```python
from build123d import *

# Parameters (mm, degrees)
SKETCH1_R           = 33.5
SKETCH1_R_2         = 4
BOSS_EXTRUDE1_DEPTH = 12
CUT_EXTRUDE1_DEPTH  = 6
SKETCH3_R           = 26
SKETCH3_R_2         = 10.5
CUT_EXTRUDE2_DEPTH  = 3
CUT_EXTRUDE3_START  = -3
SKETCH4_R           = 26
SKETCH4_R_2         = 10.5
CUT_EXTRUDE3_DEPTH  = 3
SKETCH5_R           = 2.25
SKETCH5_R_2         = 3.25
CUT_EXTRUDE4_DEPTH  = 10
CIRPATTERN1_COUNT   = 13


with BuildPart() as part:
    # Sketch1 → Boss-Extrude1 (new body)
    with BuildSketch(Plane.XY):
        Circle(SKETCH1_R)
        Circle(SKETCH1_R_2, mode=Mode.SUBTRACT)
    extrude(amount=BOSS_EXTRUDE1_DEPTH)

    # Sketch2 → Cut-Extrude1 (cut)
    with BuildSketch(Plane.XY.offset(12)):
        Polygon((7.216878365, 0), (3.608439182, 6.25), (-3.608439182, 6.25), (-7.216878365, 0), (-3.608439182, -6.25), (3.608439182, -6.25), align=None)
    extrude(amount=-CUT_EXTRUDE1_DEPTH, mode=Mode.SUBTRACT)

    # Sketch3 → Cut-Extrude2 (cut)
    with BuildSketch(Plane.XY.offset(12)):
        Circle(SKETCH3_R)
        Circle(SKETCH3_R_2, mode=Mode.SUBTRACT)
    extrude(amount=-CUT_EXTRUDE2_DEPTH, mode=Mode.SUBTRACT)

    # Sketch4 → Cut-Extrude3 (cut)
    with BuildSketch(Plane(origin=(0, 0, 0), x_dir=(-1, 0, 0), z_dir=(0, 0, -1)).offset(CUT_EXTRUDE3_START)):
        with Locations(Location((0, 0, 0), (0, 0, 180))):
            Circle(SKETCH4_R)
        with Locations(Location((0, 0, 0), (0, 0, 180))):
            Circle(SKETCH4_R_2, mode=Mode.SUBTRACT)
    extrude(amount=CUT_EXTRUDE3_DEPTH, mode=Mode.SUBTRACT)

    # Sketch5 → Cut-Extrude4 (cut)
    with BuildSketch(Plane.XY.offset(9)):
        with Locations((13.82072024, 0)):
            Circle(SKETCH5_R)
        with Locations((20.783512616, 4.875399709)):
            Circle(SKETCH5_R_2)
    cut_extrude4 = extrude(amount=-CUT_EXTRUDE4_DEPTH, mode=Mode.SUBTRACT)

    # CirPattern1: Cut-Extrude4 ×13 about axis
    cirpattern1_axis = Axis((0, 0, 0), (0, 0, 1))
    for i in range(1, CIRPATTERN1_COUNT):
        add(cut_extrude4.rotate(cirpattern1_axis, i * 360 / CIRPATTERN1_COUNT), mode=Mode.SUBTRACT)


solid = part.part
```
Source: CAD feature listing. Evaluate the final solid. Frame: model axes, mm. A direction names the side the tool comes from. Round coordinates to 2 decimals unless told otherwise and drop trailing zeros. Loops run counter-clockwise (first coordinate to the right, second up) from the corner with the lowest first, then second, coordinate; pieces in that order, holes last. Notation, with made-up numbers: M -19,27.5 L 16,27.5 A26 ccw 16,53.5 Z; hole C 28,-24.75 d9. An arc over 180 degrees is marked long. Use a Markdown table: item, result. Add a question column.
1. Cut plane B-B, the plane y = -22.5. Output: boundary loops of the cut face in (x, z).
2. Contact query for flat-ended pins moving along their axis: pin 1 (3 mm diameter, centred on y = 8, z = 4, fed in from +X); pin 2 (1 mm diameter, centred on x = 5.5, z = 8, fed in from +Y); pin 3 (5 mm diameter, centred on x = 12.24, y = -6.42, fed in from -Z). Output: stop coordinate, or through.
3. Pull-direction query (X, two-part tool) for faces 3 (the flat face through (17, -20, 12)), 4 (the flat face through (-5.387, 3.169, 9.042)); classes: +X half, -X half, draft (parallel to the pull), parting line (faces both ways), or undercut.
4. Ray query, line 1 along Y through (x, z) = (-21, 8); line 2 along X through (y, z) = (8.5, 10); line 3 along Y through (x, z) = (6, 7.25). Return the intervals inside material, ascending. Write a range as [from, to].
5. Cut plane A-A, the plane z = 5. State how many separate pieces and enclosed holes the cut face has, and give its area (3 significant figures).
6. Set-up query: faces 1 (the cylindrical face through (-2.998, -24.406, 6.042)), 2 (the flat face through (3, 3, 6)). Return all of +Z, -Z, +X, -X, +Y, -Y with unobstructed straight access to the full face (end or side cutting, diameter ignored); none if empty.
Solution:
| question | item | result |
|---|---|---|
| 1 | outline | M -24.82,0 L -13.03,0 L -13.03,3 L -5.77,3 L -5.77,9 L -13.03,9 L -13.03,12 L -24.82,12 Z; M 0.15,3 L 5.22,3 L 5.22,9 L 0.15,9 Z; M 9.47,3 L 13.03,3 L 13.03,0 L 24.82,0 L 24.82,12 L 13.03,12 L 13.03,9 L 9.47,9 Z |
| 2 | pin 1 | stops at x = 32.86 |
| 2 | pin 2 | stops at y = 33.12 |
| 2 | pin 3 | stops at z = 3 |
| 3 | face 3 | draft |
| 3 | face 4 | undercut |
| 4 | line 1 | y = [-26.1, -12.28], [-7.14, -2.99], [3.47, 7.75], [12.52, 26.1] |
| 4 | line 2 | x = [-32.4, -24.57], [-6.16, 6.16], [24.57, 32.4] |
| 4 | line 3 | y = [-32.96, -23], [-17.09, -12.65], [-10.1, -2.11], [2.11, 10.1], [12.65, 17.16], [22.58, 32.96] |
| 5 | separate pieces | 1 |
| 5 | enclosed holes | 27 |
| 5 | area | 2,840 mm2 |
| 6 | face 1 | +Z, -Z |
| 6 | face 2 | +Z |
